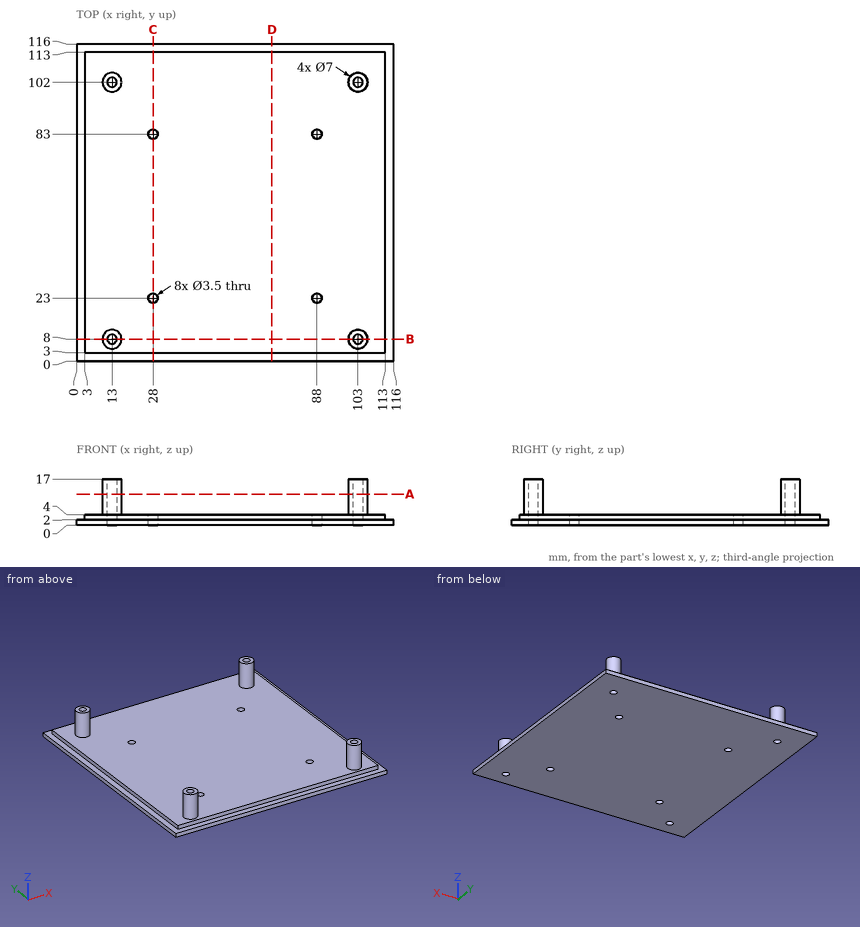
Answer from the drawing. Dimensions are ordinates in mm from the lowest x, y and z of the part. Coordinates: 2 decimals unless noted, no trailing zeros. Loops run counter-clockwise (first coordinate to the right, second up) from the corner with the lowest first, then second, coordinate; pieces in that order, holes last.
1) Section C-C (x = 28) is taken. Give the vertices of the cut face in (y, z).
Results:
outline: (0, 0) - (21.25, 0) - (21.25, 4) - (3, 4) - (3, 2) - (0, 2) - close; (24.75, 0) - (81.25, 0) - (81.25, 4) - (24.75, 4) - close; (84.75, 0) - (116, 0) - (116, 2) - (113, 2) - (113, 4) - (84.75, 4) - close
2) Section A-A (z = 11.5) is taken. Give the vertices of the cut face in (x, y).
Results:
outline: circle Ø7 at (13, 8); circle Ø7 at (13, 102); circle Ø7 at (103, 8); circle Ø7 at (103, 102); hole circle Ø3.5 at (13, 8); hole circle Ø3.5 at (13, 102); hole circle Ø3.5 at (103, 8); hole circle Ø3.5 at (103, 102)
3) Flat-ended cylindrical pins translate along their axes: pin 1 (3 mm diameter, centred on x = 13, y = 8, fed in from +Z); pin 2 (2 mm diameter, centred on x = 75.5, z = 2.5, fed in from -Y); pin 3 (5.5 mm diameter, centred on x = 28, y = 83, fed in from +Z); pin 4 (1 mm diameter, centred on y = 73.5, z = 3.5, fed in from -X). Find the tip coordinate at first contact, or state that the pin passes through.
Results:
pin 1: passes through
pin 2: stops at y = 0
pin 3: stops at z = 4
pin 4: stops at x = 3
4) Consider probe 1 along Y at (x, z) = (13, 12.25); probe 2 along X at (y, z) = (23, 1.2); probe 3 along Y at (x, z) = (88, 2.1). Determine where each line is inside the solid, lowest interval first.
Results:
probe 1: y = 4.5 to 6.25, 9.75 to 11.5, 98.5 to 100.25, 103.75 to 105.5
probe 2: x = 0 to 26.25, 29.75 to 86.25, 89.75 to 116
probe 3: y = 3 to 21.25, 24.75 to 81.25, 84.75 to 113
5) Section D-D (x = 71.5) is taken. Give the vertices of the cut face in (y, z), plus the area to 3 significant figures.
Results:
outline: (0, 0) - (116, 0) - (116, 2) - (113, 2) - (113, 4) - (3, 4) - (3, 2) - (0, 2) - close
area: 452 mm2
6) Section B-B (y = 8) is taken. Give the vertices of the cut face in (x, z), plus the area to 3 significant figures.
Results:
outline: (0, 0) - (11.25, 0) - (11.25, 17) - (9.5, 17) - (9.5, 4) - (3, 4) - (3, 2) - (0, 2) - close; (14.75, 0) - (101.25, 0) - (101.25, 17) - (99.5, 17) - (99.5, 4) - (16.5, 4) - (16.5, 17) - (14.75, 17) - close; (104.75, 0) - (116, 0) - (116, 2) - (113, 2) - (113, 4) - (106.5, 4) - (106.5, 17) - (104.75, 17) - close
area: 515 mm2
